Autodesk Inventor part; units mm, degrees
ref_plane "YZ Plane" through (0, 0, 0) normal (1, 0, 0) x (0, 1, 0)
ref_plane "XZ Plane" through (0, 0, 0) normal (0, 1, 0) x (-1, 0, 0)
ref_plane "XY Plane" through (0, 0, 0) normal (0, 0, 1) x (1, 0, 0)
sketch "Sketch1" plane through (0, 0, 0) normal (0, 0, 1) x (1, 0, 0)
  circle A0 centre (0, 0) radius 38.1
  circle A1 centre (0, 0) radius 27.94 construction
  circle A2 centre (0, 27.94) radius 3
  circle A3 centre (0, 0) radius 27.94 construction
  circle A4 centre (-19.7566, 19.7566) radius 3
  circle A5 centre (0, 0) radius 27.94 construction
  circle A6 centre (-27.94, 0) radius 3
  circle A7 centre (0, 0) radius 27.94 construction
  circle A8 centre (-19.7566, -19.7566) radius 3
  circle A9 centre (0, 0) radius 27.94 construction
  circle A10 centre (0, -27.94) radius 3
  circle A11 centre (0, 0) radius 27.94 construction
  circle A12 centre (19.7566, -19.7566) radius 3
  circle A13 centre (0, 0) radius 27.94 construction
  circle A14 centre (27.94, 0) radius 3
  circle A15 centre (0, 0) radius 27.94 construction
  circle A16 centre (19.7566, 19.7566) radius 3
  dimension "d1" = 55.88
  dimension "d0" = 76.2
  dimension "d2" = 6
  dimension "d5" = 360
extrude "Extrusion1" add sketch "Sketch1" along normal blind 6.35
sketch "Sketch2" plane through (0, 0, 6.35) normal (0, 0, 1) x (1, 0, 0)
  circle A0 centre (0, 0) radius 6.35
  dimension "d9" = 12.7
extrude "Extrusion2" add sketch "Sketch2" along normal blind 25.4
sketch "Sketch3" plane through (0, 0, 31.75) normal (0, 0, 1) x (1, 0, 0)
  arc A0 (-6.35, 0) -> (6.35, 0) centre (0, 0) ccw
  line L0 (6.35, 0) -> (6.35, 76.2397)
  line L1 (-6.35, 0) -> (-6.35, 76.2397)
  arc A1 (6.35, 76.2397) -> (-6.35, 76.2397) centre (0, 76.2397) ccw
extrude "Extrusion3" add sketch "Sketch3" along normal blind 8.382
properties part number "pin holder"
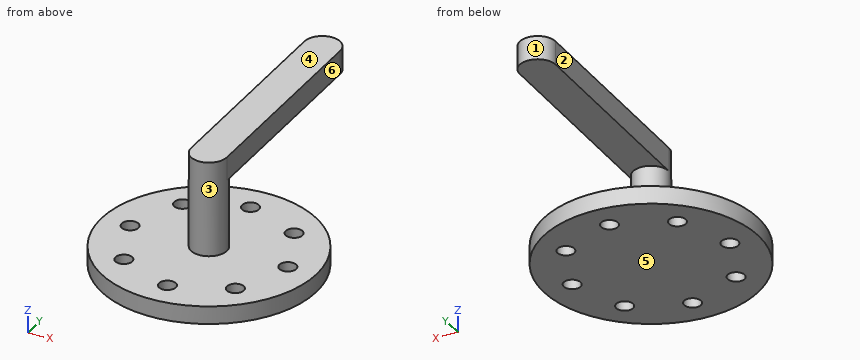
Geometry check sheet. Reference: the model listing, model coordinates, mm. Face numbers are marked on the shaded views. A direction names the side the tool comes from. Coordinates: 2 decimals unless noted, no trailing zeros. Write each loop counter-clockwise with the first axis right and the second up, starting at its lowest first coordinate (ties: lowest second). Pieces come first, ordered by that corner, then holes. Notation, with made-up numbers: M 49,-13 L 105,-13 A24 ccw 105,9 Z; hole C 41.25,17 d11. An arc over 180 degrees is marked long. Answer as a JSON object with one key per item and string values.
1. Tool access check on the marked faces 1 and 2. Record the directions out of +Z, -Z, +X, -X, +Y, -Y that give a thin tool (end or side, any length) a straight path to the whole face; none if there is none.
Answers below:
{"face 1": "+Z, -Z, +Y", "face 2": "+Z, -X, +Y, -Y"}
2. Draft check along Z on the marked faces 3, 4, 5 and 6. Enter one of: released by +Z, released by -Z, zero draft, split by the parting line, or undercut.
Answers below:
{"face 3": "undercut", "face 4": "released by +Z", "face 5": "released by -Z", "face 6": "zero draft"}
3. Scan lines: L1, parallel to Y at x = 0, z = 4; L2, parallel to Z at x = -4, y = 21.5; L3, parallel to Z at x = 24.5, y = 14.5. Record each from-to range of solid material in increasing order.
Answers below:
{"L1": "y = -38.1 to -30.94, -24.94 to 24.94, 30.94 to 38.1", "L2": "z = 0 to 6.35, 31.75 to 40.13", "L3": "z = 0 to 6.35"}
4. Section check A-A, the plane x = 0. Enter the section's corners in (y, z), plus the area to 3 significant figures.
Answers below:
{"outline": "M -38.1,0 L -30.94,0 L -30.94,6.35 L -38.1,6.35 Z; M -24.94,0 L 24.94,0 L 24.94,6.35 L 6.35,6.35 L 6.35,31.75 L 82.59,31.75 L 82.59,40.13 L -6.35,40.13 L -6.35,6.35 L -24.94,6.35 Z; M 30.94,0 L 38.1,0 L 38.1,6.35 L 30.94,6.35 Z", "area": "1,480 mm²"}
5. Section check C-C, the plane y = -27.94. Enter the section's corners in (x, z).
Answers below:
{"outline": "M -25.9,0 L -3,0 L -3,6.35 L -25.9,6.35 Z; M 3,0 L 25.9,0 L 25.9,6.35 L 3,6.35 Z"}
6. Section check B-B, the plane y = 27.94. Enter the section's corners in (x, z).
Answers below:
{"outline": "M -25.9,0 L -3,0 L -3,6.35 L -25.9,6.35 Z; M -6.35,31.75 L 6.35,31.75 L 6.35,40.13 L -6.35,40.13 Z; M 3,0 L 25.9,0 L 25.9,6.35 L 3,6.35 Z"}
7. Go/stop test with flat-tipped pins: pin 1 Ø4 at (x, z) = (-9.5, 22) entering from +Y; pin 2 Ø8 at (x, y) = (24, -18) entering from +Z; pin 3 Ø10 at (x, z) = (5, 23.5) entering from -Y; pin 4 Ø10 at (x, z) = (21, 7.5) entering from +Y. Record where each tip stops, or that it passes through.
Answers below:
{"pin 1": "passes through", "pin 2": "stops at z = 6.35", "pin 3": "stops at y = -6.35", "pin 4": "stops at y = 34.52"}
